Autodesk Inventor part; units mm, degrees
ref_plane "YZ Plane" through (0, 0, 0) normal (1, 0, 0) x (0, 1, 0)
ref_plane "XZ Plane" through (0, 0, 0) normal (0, 1, 0) x (-1, 0, 0)
ref_plane "XY Plane" through (0, 0, 0) normal (0, 0, 1) x (1, 0, 0)
sketch "スケッチ1" plane through (0, 0, 0) normal (0, 0, 1) x (1, 0, 0)
  circle A0 centre (0, 0) radius 2
  dimension "d0" = 4
extrude "押し出し1" add sketch "スケッチ1" along normal blind 6
sketch "スケッチ2" plane through (0, 0, 6) normal (0, 0, 1) x (1, 0, 0)
  circle A0 centre (0, 0) radius 2
  circle A1 centre (0, 0) radius 4
  dimension "d3" = 8
extrude "押し出し2" add sketch "スケッチ2" along normal blind 2.3 contours A0 | A1
thread "ねじ1"
chamfer "面取り1" distance 2 angle 45 1 edges at (-4, 0, 6)
sketch "スケッチ4" plane through (0, 0, 0) normal (0, 0, -1) x (-1, 0, 0)
  circle A0 centre (0, 0) radius 2
extrude "押し出し4" add sketch "スケッチ4" along normal blind 11.7
sketch "スケッチ5" plane through (0, 0, 8.3) normal (0, 0, 1) x (1, 0, 0)
  line L0 (-1.5, 0.866) -> (0, 1.7321)
  line L1 (0, 1.7321) -> (1.5, 0.866)
  line L2 (1.5, 0.866) -> (1.5, -0.866)
  line L3 (1.5, -0.866) -> (0, -1.7321)
  line L4 (0, -1.7321) -> (-1.5, -0.866)
  line L5 (-1.5, -0.866) -> (-1.5, 0.866)
  point P0 (0, 0)
  point P1 (0, 0)
  point P2 (-1.5, 0)
  dimension "d16" = 3
extrude "押し出し5" cut sketch "スケッチ5" against normal blind 2
properties part number "SB　M4 20mm 皿ネジ" material "Stainless Steel, 440C"
For this review, take the finished solid that the model builds, in its own axes (mm). A direction names the side the tool comes from. Give positions to 0.01 mm unless a question says otherwise; leave off trailing zeros. Loops run counter-clockwise (first coordinate to the right, second up) from the corner with the lowest first, then second, coordinate; pieces in that order, holes last. Notation, with made-up numbers: M -37,-4.5 L -13,-4.5 A28 cw -13,23.5 Z; hole C -12.75,51.25 d5. An arc over 180 degrees is marked long. Answer as a JSON object with one key per item and string values. Group by question number.
Q1. Mouldability with a two-part tool opening along X and no side actions: class faces 1 (the flat face through (0, 0, 6.3)), 2 (the flat face through (0, 0, -11.7)), 3 (the conical face through (-0.46, -2.08, 6.13)) as +X half, -X half, draft (parallel to the pull), parting line (faces both ways), or undercut.
Q2. Add section B-B on z = -2. Give the boundary of the cut face in (x, y).
Q3. Insertion check: P1, Ø0.9, axis at y = 0, z = 7.5, coming from the -X side; P2, Ø1, axis at y = -1, z = 2.5, coming from the -X side; P3, Ø1.5, axis at x = 1.5, z = -4.5, coming from the +Y side. Each pin has a flat end and moves straight along its axis. Give the tip position at first contact, or say it passes through.
Q4. Tool access review of faces 4 (the flat face through (2, 0, 8.3)), 5 (the flat face through (0.74, 1.305, 7.314)): name each direction out of +Z, -Z, +X, -X, +Y, -Y from which nothing blocks a thin tool from reaching the whole face with its end or side.
Q5. For probe 1 along X at (y, z) = (-1.25, 6.5); probe 2 along Y at (x, z) = (0.5, 5.75); probe 3 along Z at (x, y) = (0.75, -3.5), list the stretches that pass through material, from the lowest coordinate up. Write a range as [from, to].
Checked values:
{
 "1": {"face 1": "undercut", "face 2": "draft", "face 3": "parting line"},
 "2": {"outline": "C 0,0 d4"},
 "3": {"P1": "x = -3.95", "P2": "x = -1.94", "P3": "y = 1.85"},
 "4": {"face 4": "+Z, +X, -X, +Y, -Y", "face 5": "+Z"},
 "5": {"probe 1": "[-2.17, -0.83], [0.83, 2.17]", "probe 2": "[-1.94, 1.94]", "probe 3": "[7.58, 8.3]"}
}
